Autodesk Inventor part; units mm, degrees
ref_plane "YZ Plane" through (0, 0, 0) normal (1, 0, 0) x (0, 1, 0)
ref_plane "XZ Plane" through (0, 0, 0) normal (0, 1, 0) x (-1, 0, 0)
ref_plane "XY Plane" through (0, 0, 0) normal (0, 0, 1) x (1, 0, 0)
sketch "Sketch3" plane through (0, 0, 0) normal (0, 0, 1) x (1, 0, 0)
  circle A0 centre (0, 0) radius 2
  line L0 (1.0225, 0.5903) -> (1.0225, -0.5903)
  line L1 (1.0225, -0.5903) -> (0, -1.1807)
  line L2 (0, -1.1807) -> (-1.0225, -0.5903)
  line L3 (-1.0225, -0.5903) -> (-1.0225, 0.5903)
  line L4 (-1.0225, 0.5903) -> (0, 1.1807)
  line L5 (0, 1.1807) -> (1.0225, 0.5903)
  line L6 (0, 0) -> (0, 1.1807) construction
  dimension "HexWidth" = 2.045
sketch "Sketch2" plane through (0, 0, 0) normal (0, 0, 1) x (1, 0, 0)
  circle A0 centre (0, 0) radius 2
  dimension "Diam" = 4
extrude "Extrusion2" add sketch "Sketch2" against normal blind 6
thread "Thread1"
extrude "Extrusion3" cut sketch "Sketch3" against normal blind 2.5 contours L0 L1 L2 L3 L4 L5
chamfer "Chamfer2" distance 0.75 angle 45 1 edges at (-2, 0, -6)
chamfer "Chamfer3" distance 0.1875 angle 45 1 edges at (-2, 0, 0)
sketch "Sketch4" plane through (0, 0, -6) normal (0, 0, -1) x (-1, 0, 0)
  circle A0 centre (0, 0) radius 1.8125
hole "Cup_Point_Hole1" at (0, 0, -6) direction (0, 0, 1) diameter 2.4999 depth 0.001 tip angle 118
equation "\"d8\" = -0.5 * CupPointDiam + 0.5 * Diam"
equation "\"d11\" = 0.25 * d8"
equation "\"CupPointDiam\" = 2.5"
properties part number "SCREW,SET,CUP POINT,M4X0.7X6MM" material "Steel, MS"
Part model, mm, in its own coordinate system. A direction names the side the tool comes from. Round coordinates to 2 decimals unless told otherwise and drop trailing zeros. Loops run counter-clockwise (first coordinate to the right, second up) from the corner with the lowest first, then second, coordinate; pieces in that order, holes last.
1. Drill centre lines: line 1 along X through (y, z) = (-0.05, -5.4); line 2 along Y through (x, z) = (0.7, -1.5); line 3 along Z through (x, y) = (-0.5, -0.6). Where is each one in solid material? Low to high.
Solutions:
line 1: x = -1.85 to -0.25, 0.25 to 1.85
line 2: y = -1.87 to -0.78, 0.78 to 1.87
line 3: z = -5.72 to -2.5
2. Slice it at A-A (z = -1.15). Give the cut face in (x, y).
Solutions:
outline: circle Ø4 at (0, 0); hole (-1.02, -0.59) - (0, -1.18) - (1.02, -0.59) - (1.02, 0.59) - (0, 1.18) - (-1.02, 0.59) - close
3. Flat gauge pin, fed straight in: pin 1 (0.6 mm diameter, centred on x = 0.5, y = -0.5, fed in from +Z). Where does the tip first touch, or does it go through?
Solutions:
pin 1: stops at z = -2.5
4. 3-axis set-ups, long thin cutter, end or side, ignore diameter. For faces 1 (the face through (0, -2, -3)), 2 (the face through (0.52, -0.88, -1.23)): which of +Z, -Z, +X, -X, +Y, -Y reach the whole face in a straight line?
Solutions:
face 1: +Z, -Z
face 2: +Z
5. Slice it at B-B (z = -4.4). Give the cut face in (x, y), and give its area (3 significant figures).
Solutions:
outline: circle Ø4 at (0, 0)
area: 12.6 mm2
